Read the model definition and answer for the solid it produces. Units are mm, in the model's axes. A direction names the side the tool comes from. Round coordinates to 2 decimals unless told otherwise and drop trailing zeros. Write each loop counter-clockwise with the first axis right and the second up, starting at its lowest first coordinate (ties: lowest second). Pieces come first, ordered by that corner, then holes. Notation, with made-up numbers: (-20, 9.25) - (34, 9.25) arc R31 cw to (34, 45.25) - close; hole circle Ø6 at (33.5, 75.5). An arc over 180 degrees is marked (long way). Use one line per item in the form item = value. Start each with the question number.
1) Each of these flat-tipped pins is pushed along its axis until it touches: pin 1 (2 mm diameter, centred on y = 116.5, z = -4.5, fed in from +X); pin 2 (10 mm diameter, centred on x = -1, y = 71.5, fed in from +Z); pin 3 (1.5 mm diameter, centred on x = -6.5, y = 19.5, fed in from -Z). Where does it stop, or does it pass through?
2) The part is cut by section D-D, the plane z = 10.25. Give the vertices of the cut face in (x, y), plus the area to 3 significant figures.
3) The part is cut by section B-B, the plane x = 0. Give the vertices of the cut face in (y, z), plus the area to 3 significant figures.
4) For faces 1 (the face through (3.604, 1.479, 11.446)), 2 (the face through (2, 140, 5)), determine the directions among +Z, -Z, +X, -X, +Y, -Y from which every point of the face is accessible in a straight line to the end or side of a thin tool.
5) The part is cut by section C-C, the plane y = 28.5. Give the vertices of the cut face in (x, z).
6) Consider line 1 along Y through (x, z) = (7, -1.25); line 2 along X through (y, z) = (134, 0); line 3 along Y through (x, z) = (1, -6.5). Determine where each line is inside the solid, lowest interval first. Write a range as from..to.
7) The part is cut by section A-A, the plane z = 0. Give the vertices of the cut face in (x, y).
from build123d import *

# Parameters (mm, degrees)
SKETCH1_R         = 12
FOOT_FLANGE_DEPTH = 3
SKETCH2_R         = 7
LEG_DEPTH         = 140
SPIGOT_START      = 140
SKETCH3_R         = 4.8
SPIGOT_DEPTH      = 1.8


with BuildPart() as part:
    # Sketch1 → Foot_Flange (new body)
    with BuildSketch(Plane(origin=(0, 0, 0), x_dir=(1, 0, 0), z_dir=(0, 1, 0))):
        with Locations(Location((0, 0, 0), (0, 0, 270))):
            Circle(SKETCH1_R)
    extrude(amount=FOOT_FLANGE_DEPTH)

    # Sketch2 → Leg (add)
    with BuildSketch(Plane(origin=(0, 0, 0), x_dir=(1, 0, 0), z_dir=(0, 1, 0))):
        with Locations(Location((0, 0, 0), (0, 0, 270))):
            Circle(SKETCH2_R)
    extrude(amount=LEG_DEPTH)

    # Sketch3 → Spigot (add)
    with BuildSketch(Plane(origin=(0, 0, 0), x_dir=(1, 0, 0), z_dir=(0, 1, 0)).offset(SPIGOT_START)):
        with Locations(Location((0, 0, 0), (0, 0, 270))):
            Circle(SKETCH3_R)
    extrude(amount=SPIGOT_DEPTH)


solid = part.part
Geometry results:
q1.pin_1 = 6.06
q1.pin_2 = 7
q1.pin_3 = -3.99
q2.outline = (-6.24, 0) - (6.24, 0) - (6.24, 3) - (-6.24, 3) - close
q2.area = 37.4 mm2
q3.outline = (0, -12) - (3, -12) - (3, -7) - (140, -7) - (140, -4.8) - (141.8, -4.8) - (141.8, 4.8) - (140, 4.8) - (140, 7) - (3, 7) - (3, 12) - (0, 12) - close
q3.area = 2,010 mm2
q4.face_1 = +Y, -Y
q4.face_2 = +Y
q5.outline = circle Ø14 at (0, 0)
q6.line_1 = 0..3
q6.line_2 = -7..7
q6.line_3 = 0..140
q7.outline = (-12, 0) - (12, 0) - (12, 3) - (7, 3) - (7, 140) - (4.8, 140) - (4.8, 141.8) - (-4.8, 141.8) - (-4.8, 140) - (-7, 140) - (-7, 3) - (-12, 3) - close
